The listing builds one solid part. Answer for the finished solid, in the listing's coordinates (mm). A direction names the side the tool comes from. Round coordinates to 2 decimals unless told otherwise and drop trailing zeros. Loops run counter-clockwise (first coordinate to the right, second up) from the corner with the lowest first, then second, coordinate; pieces in that order, holes last. Notation, with made-up numbers: (49.25, -31.5) - (97.25, -31.5) arc R9 ccw to (97.25, -15.5) - close; hole circle Ø11 at (-9, 15). An arc over 180 degrees is marked (long way). One line per question, with ' | ' between items. Start each with the question number.
from build123d import *

# Parameters (mm, degrees)
SKETCH1_W           = 25
SKETCH1_H           = 8
SKETCH1_R           = 1.3
BOSS_EXTRUDE1_DEPTH = 3.5
FILLET1_R           = 4
SKETCH3_R           = 1.3
CUT_EXTRUDE6_DEPTH  = 9
SKETCH5_R           = 2.5
CUT_EXTRUDE7_DEPTH  = 3


with BuildPart() as part:
    # Sketch1 → Boss-Extrude1 (new body, symmetric)
    with BuildSketch(Plane(origin=(0, 0, 0), x_dir=(0, 0, -1), z_dir=(1, 0, 0))):
        with Locations((-8.5, 0)):
            Rectangle(SKETCH1_W, SKETCH1_H)
        Circle(SKETCH1_R, mode=Mode.SUBTRACT)
    extrude(amount=BOSS_EXTRUDE1_DEPTH, both=True)

    # Fillet1
    fillet1_edges = [part.edges().sort_by_distance(p)[0] for p in [
        (0, -4, -4),
    ]]
    fillet(fillet1_edges, radius=FILLET1_R)

    # Sketch3 → Cut-Extrude6 (cut, through all)
    with BuildSketch(Plane(origin=(0, 4, 0), x_dir=(1, 0, 0), z_dir=(0, 1, 0))):
        with Locations((0, -6)):
            Circle(SKETCH3_R)
        with Locations((0, -16)):
            Circle(SKETCH3_R)
    extrude(amount=-CUT_EXTRUDE6_DEPTH, mode=Mode.SUBTRACT)

    # Sketch5 → Cut-Extrude7 (cut)
    with BuildSketch(Plane.XZ.offset(4)):
        with Locations((0, 16)):
            Circle(SKETCH5_R)
        with Locations((0, 6)):
            Circle(SKETCH5_R)
    extrude(amount=-CUT_EXTRUDE7_DEPTH, mode=Mode.SUBTRACT)


solid = part.part
(1) Determine the mould class of faces 3 (the flat face through (0, 2, -4)), 4 (the cylindrical face through (-0.33, -2.52, 8.48)), 5 (the cylindrical face through (-0.54, -2.52, 13.56)), 6 (the flat face through (3.5, 0, 9)) for opening direction X: pulls with the +X half, pulls with the -X half, needs draft (parallel to the pull), parting line crosses it, or undercut.
(2) Each of these flat-tipped pins is pushed along its axis until it touches: P1, Ø1, axis at x = -2, y = -1, coming from the -Z side; P2, Ø2, axis at y = 0, z = 0, coming from the -X side; P3, Ø3, axis at x = 0, z = 16, coming from the -Y side; P4, Ø4, axis at x = -0.5, z = 16.5, coming from the +Y side. Where does it stop, or does it pass through?
(3) Find section C-C on y = -0.75. Write down the section's boundary in (x, z).
(4) A tool of negligible diameter and unlimited length cuts with its end or side. For faces 1 (the flat face through (1.1, -1, 4.9)), 2 (the flat face through (-3.5, 0, 9)), from which of +Z, -Z, +X, -X, +Y, -Y can it reach the whole face along a straight path? Write none if from no direction.
(5) Find section B-B on z = 16. Write down the section's boundary in (x, y).
(6) Consider L1, parallel to Z at x = 0, y = 1.8; L2, parallel to Z at x = -1.5, y = -1.75; L3, parallel to X at y = 1.65, z = 6. Determine where each line is inside the solid, lowest interval first.
(7) Find section D-D on x = 3. Write down the section's boundary in (y, z).
(8) Find section A-A on x = 0. Write down the section's boundary in (y, z).
Answer below:
1) face 3: needs draft | face 4: undercut | face 5: undercut | face 6: pulls with the +X half
2) P1: z = -3.97 | P2: through | P3: y = -1 | P4: y = 4
3) outline: (-3.5, -3.93) - (3.5, -3.93) - (3.5, -1.06) - (-3.5, -1.06) - close; (-3.5, 1.06) - (3.5, 1.06) - (3.5, 21) - (-3.5, 21) - close; hole circle Ø2.6 at (0, 6); hole circle Ø2.6 at (0, 16)
4) face 1: -Y | face 2: +Z, -Z, -X, +Y, -Y
5) outline: (-3.5, -4) - (-2.5, -4) - (-2.5, -1) - (-1.3, -1) - (-1.3, 4) - (-3.5, 4) - close; (1.3, -1) - (2.5, -1) - (2.5, -4) - (3.5, -4) - (3.5, 4) - (1.3, 4) - close
6) L1: -4 to 4.7, 7.3 to 14.7, 17.3 to 21 | L2: -3.6 to 4, 8 to 14, 18 to 21 | L3: -3.5 to -1.3, 1.3 to 3.5
7) outline: (-4, 0) arc R4 ccw to (0, -4) - (4, -4) - (4, 21) - (-4, 21) - close; hole circle Ø2.6 at (0, 0)
8) outline: (-4, 0) arc R4 ccw to (0, -4) - (4, -4) - (4, 4.7) - (-1, 4.7) - (-1, 3.5) - (-4, 3.5) - close; (-4, 8.5) - (-1, 8.5) - (-1, 7.3) - (4, 7.3) - (4, 14.7) - (-1, 14.7) - (-1, 13.5) - (-4, 13.5) - close; (-4, 18.5) - (-1, 18.5) - (-1, 17.3) - (4, 17.3) - (4, 21) - (-4, 21) - close; hole circle Ø2.6 at (0, 0)
